Geometry check sheet. Reference: drawing and pictorial views, mm from the part's lowest x, y, z. A direction names the side the tool comes from. Give positions to 0.01 mm unless a question says otherwise; leave off trailing zeros. Order: outer loops, then holes, each group sorted by start corner. A loop starts at its lowest first (then second) coordinate and runs counter-clockwise, first axis right, second up. Notation, with made-up numbers: (33, 0) - (88, 0) arc R18 cw to (88, 25) - close; hole circle Ø11 at (-33, 89). An arc over 180 degrees is marked (long way). Answer in a Markdown table with one row per item.
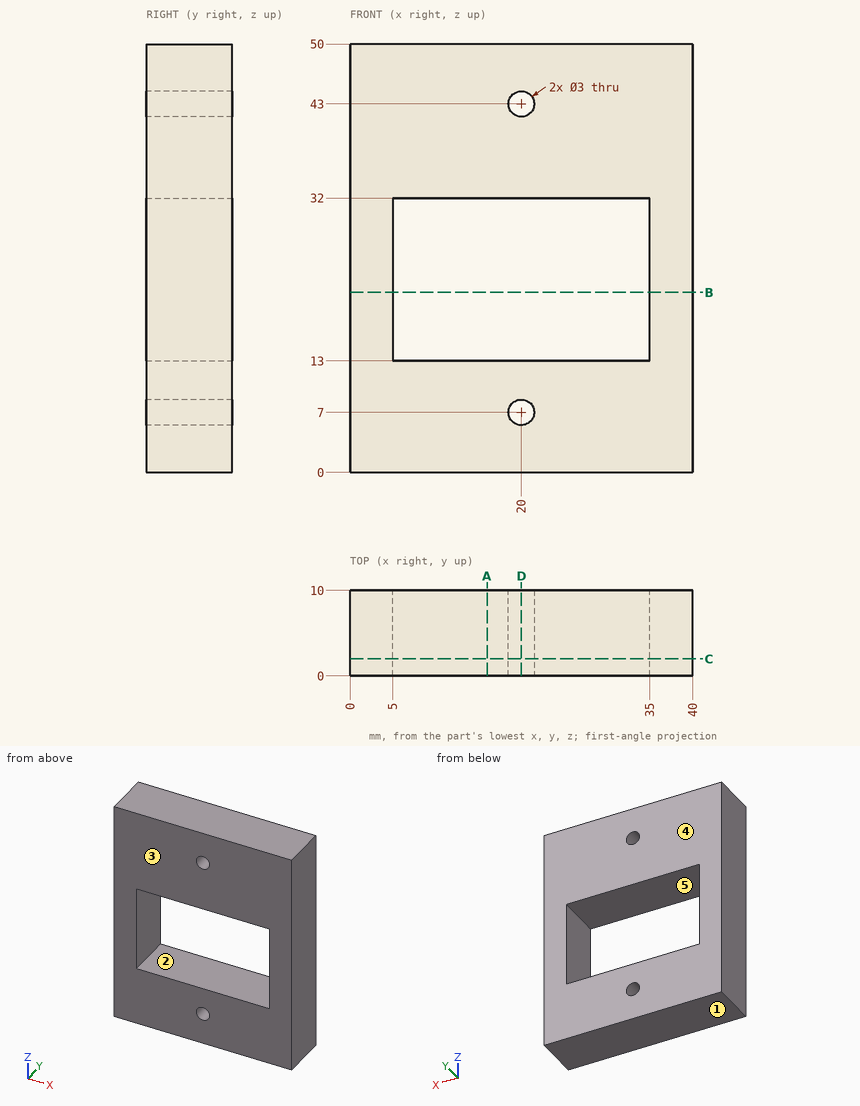
(1) Thickness scan on L1, parallel to Z at x = 20, y = 4.5; L2, parallel to Z at x = 32, y = 1; L3, parallel to X at y = 5.5, z = 26.5. Record the ranges inside material, lowest first.
Geometry says:
| item | result |
|---|---|
| L1 | 0 to 5.5, 8.5 to 13, 32 to 41.5, 44.5 to 50 |
| L2 | 0 to 13, 32 to 50 |
| L3 | 0 to 5, 35 to 40 |
(2) Access from +Z, -Z, +X, -X, +Y, -Y to the whole of each face (thin tool, end or side, straight path). Record for the marked faces 4 and 5.
Geometry says:
| item | result |
|---|---|
| face 4 | +Z, -Z, +X, -X, +Y |
| face 5 | +Y, -Y |
(3) Cross-section at C-C, the plane y = 2. Record the cut outline in (x, z).
Geometry says:
| item | result |
|---|---|
| outline | (0, 0) - (40, 0) - (40, 50) - (0, 50) - close; hole (5, 13) - (35, 13) - (35, 32) - (5, 32) - close; hole circle Ø3 at (20, 7); hole circle Ø3 at (20, 43) |
(4) Mould release check, pull along Z, two halves, no side actions. Record for the marked faces 1, 2 and 3: pulls with the +Z half, pulls with the -Z half, needs draft (parallel to the pull), parting line crosses it, or undercut.
Geometry says:
| item | result |
|---|---|
| face 1 | pulls with the -Z half |
| face 2 | undercut |
| face 3 | needs draft |
(5) Cross-section at B-B, the plane z = 21. Record the cut outline in (x, y), then the cut area to 3 significant figures.
Geometry says:
| item | result |
|---|---|
| outline | (0, 0) - (5, 0) - (5, 10) - (0, 10) - close; (35, 0) - (40, 0) - (40, 10) - (35, 10) - close |
| area | 100 mm² |
(6) Cross-section at D-D, the plane x = 20. Record the cut outline in (y, z).
Geometry says:
| item | result |
|---|---|
| outline | (0, 0) - (10, 0) - (10, 5.5) - (0, 5.5) - close; (0, 8.5) - (10, 8.5) - (10, 13) - (0, 13) - close; (0, 32) - (10, 32) - (10, 41.5) - (0, 41.5) - close; (0, 44.5) - (10, 44.5) - (10, 50) - (0, 50) - close |
(7) Cross-section at A-A, the plane x = 16. Record the cut outline in (y, z), then the cut area to 3 significant figures.
Geometry says:
| item | result |
|---|---|
| outline | (0, 0) - (10, 0) - (10, 13) - (0, 13) - close; (0, 32) - (10, 32) - (10, 50) - (0, 50) - close |
| area | 310 mm² |
